Part model, mm, in its own coordinate system. A direction names the side the tool comes from. Round coordinates to 2 decimals unless told otherwise and drop trailing zeros. Write each loop counter-clockwise with the first axis right and the second up, starting at its lowest first coordinate (ties: lowest second). Pieces come first, ordered by that corner, then holes. Notation, with made-up numbers: M 64.25,-20.5 L 106.25,-20.5 A32 ccw 106.25,10.5 Z; hole C 15,-36 d10. An arc over 180 degrees is marked long. Use a Markdown table: item, result. Add a question column.
1) Two-plate mould, pull along Z, no slides. Class faces 1 (the face through (100.487, 3.479, -4.305)), 2 (the face through (113, 2, -64)), 3 (the face through (-14.5, 35, -21)): released by +Z, released by -Z, zero draft, split by the parting line, or undercut.
2) Which spindle directions (+Z, -Z, +X, -X, +Y, -Y) get a long thin tool onto all of the face, cutting with end or side? Do faces 4 (the face through (113, 2, 18)), 5 (the face through (-1.2, 52.5, -25.5)), 6 (the face through (41.974, 0.986, -4.109)), 7 (the face through (113, 2, 29)). Say none if no direction does.
3) Slice it at B-B on z = -26.7. Write the cut outline in (x, y), plus the area to 3 significant figures.
4) Drop flat-ended pins along their axis: P1, Ø1.8, axis at x = 98.5, z = -68.5, coming from the -Y side; P2, Ø4, axis at x = 20, y = 47, coming from the +Z side; P3, Ø5.5, axis at y = 2, z = 22.5, coming from the -X side; P4, Ø1, axis at y = 20.5, z = -43.5, coming from the -X side. Give the stop position or say it passes through.
5) Wall check: probe 1 along X at (y, z) = (51, -3); probe 2 along Z at (x, y) = (99, 4.25); probe 3 along X at (y, z) = (0.55, -67.5). Give the ranges that are in metal, low to high.
6) Slice it at D-D on y = 23. Write the cut outline in (x, z).
7) Slice it at A-A on x = 10. Write the cut outline in (y, z), plus the area to 3 significant figures.
8) Slice it at C-C on x = 25. Write the cut outline in (y, z).
```python
from build123d import *

# Parameters (mm, degrees)
SKETCH_1_W               = 4
SKETCH_1_H               = 42
SKETCH_1_W_2             = 29
SKETCH_1_W_3             = 16
EXTRUDE_2_DEPTH          = 90
CUT_EXTRUDE_3_DEPTH      = 30
CUT_EXTRUDE_3_DEPTH_BACK = 1
SKETCH_1_6_W             = 29
SKETCH_1_6_H             = 42
SKETCH_7_W               = 77
SKETCH_7_H               = 115
CUT_EXTRUDE_5_DEPTH      = 85
SKETCH_8_W               = 49
SKETCH_8_H               = 42
CUT_EXTRUDE_6_DEPTH      = 55
SKETCH_11_R              = 1.5
CUT_EXTRUDE_9_DEPTH      = 6
SKETCH_14_R              = 3
CUT_EXTRUDE_11_DEPTH     = 2
SKETCH_18_W              = 49
SKETCH_18_H              = 42
EXTRUDE_3_DEPTH          = 20
SKETCH_19_W              = 29
SKETCH_19_H              = 42
CUT_EXTRUDE_14_DEPTH     = 20
SKETCH_20_R              = 1.5
CUT_EXTRUDE_15_DEPTH     = 141.289878466
SKETCH_21_R              = 2.75
CUT_EXTRUDE_16_DEPTH     = 2.5
SKETCH_25_W              = 4
SKETCH_25_H              = 42
CUT_EXTRUDE_18_DEPTH     = 20
SKETCH_26_W              = 11
SKETCH_26_H              = 11
EXTRUDE_4_DEPTH          = 5
SKETCH_28_R              = 3
CUT_EXTRUDE_19_DEPTH     = 151.639470259


with BuildPart() as part:
    # 草图1 → 凸台-拉伸2 (new body)
    with BuildSketch(Plane(origin=(0, 0, 0), x_dir=(1, 0, 0), z_dir=(0, 1, 0))):
        with Locations((-16.5, 21)):
            Rectangle(SKETCH_1_W, SKETCH_1_H)
        with Locations((0, 21)):
            Rectangle(SKETCH_1_W_2, SKETCH_1_H)
        with Locations((22.5, 21)):
            Rectangle(SKETCH_1_W_3, SKETCH_1_H)
        with Locations((32.5, 21)):
            Rectangle(SKETCH_1_W, SKETCH_1_H)
        Polygon((30.5, 75), (30.5, 42), (34.5, 42), (34.5, 0), (30.5, 0), (30.5, -40), (107.5, -40), (107.5, 75), align=None)
    extrude(amount=EXTRUDE_2_DEPTH)

    # 草图1<6> → 切除-拉伸3 (cut, two sides: drawn at the far end of the back side and taken through both)
    with BuildSketch(Plane(origin=(0, 0, 0), x_dir=(1, 0, 0), z_dir=(0, 1, 0)).offset(-CUT_EXTRUDE_3_DEPTH_BACK)):
        with Locations((0, 21)):
            Rectangle(SKETCH_1_6_W, SKETCH_1_6_H)
    extrude(amount=CUT_EXTRUDE_3_DEPTH + CUT_EXTRUDE_3_DEPTH_BACK, mode=Mode.SUBTRACT)

    # 草图7 → 切除-拉伸5 (cut)
    with BuildSketch(Plane(origin=(0, 90, 0), x_dir=(1, 0, 0), z_dir=(0, 1, 0))):
        with Locations((69, 17.5)):
            Rectangle(SKETCH_7_W, SKETCH_7_H)
    extrude(amount=-CUT_EXTRUDE_5_DEPTH, mode=Mode.SUBTRACT)

    # 草图8 → 切除-拉伸6 (cut)
    with BuildSketch(Plane(origin=(0, 90, 0), x_dir=(1, 0, 0), z_dir=(0, 1, 0))):
        with Locations((6, 21)):
            Rectangle(SKETCH_8_W, SKETCH_8_H)
    extrude(amount=-CUT_EXTRUDE_6_DEPTH, mode=Mode.SUBTRACT)

    # 草图11 → 切除-拉伸9 (cut)
    with BuildSketch(Plane.XZ):
        with Locations(Location((39, 33, 0), (0, 0, 270))):
            Circle(SKETCH_11_R)
        with Locations(Location((99, 33, 0), (0, 0, 270))):
            Circle(SKETCH_11_R)
        with Locations(Location((39, -4.5, 0), (0, 0, 270))):
            Circle(SKETCH_11_R)
        with Locations(Location((99, -4.5, 0), (0, 0, 270))):
            Circle(SKETCH_11_R)
        with Locations(Location((99, -67.5, 0), (0, 0, 270))):
            Circle(SKETCH_11_R)
        with Locations(Location((39, -67.5, 0), (0, 0, 270))):
            Circle(SKETCH_11_R)
    extrude(amount=-CUT_EXTRUDE_9_DEPTH, mode=Mode.SUBTRACT)

    # 草图14 → 切除-拉伸11 (cut)
    with BuildSketch(Plane.XZ):
        with Locations(Location((39, 33, 0), (0, 0, 270))):
            Circle(SKETCH_14_R)
        with Locations(Location((99, 33, 0), (0, 0, 270))):
            Circle(SKETCH_14_R)
        with Locations(Location((39, -4.5, 0), (0, 0, 270))):
            Circle(SKETCH_14_R)
        with Locations(Location((99, -4.5, 0), (0, 0, 270))):
            Circle(SKETCH_14_R)
        with Locations(Location((39, -67.5, 0), (0, 0, 270))):
            Circle(SKETCH_14_R)
        with Locations(Location((99, -67.5, 0), (0, 0, 270))):
            Circle(SKETCH_14_R)
    extrude(amount=-CUT_EXTRUDE_11_DEPTH, mode=Mode.SUBTRACT)

    # 草图18 → 凸台-拉伸3 (add)
    with BuildSketch(Plane(origin=(0, 35, 0), x_dir=(1, 0, 0), z_dir=(0, 1, 0))):
        with Locations((6, 21)):
            Rectangle(SKETCH_18_W, SKETCH_18_H)
    extrude(amount=EXTRUDE_3_DEPTH)

    # 草图19 → 切除-拉伸14 (cut)
    with BuildSketch(Plane.XZ.offset(-30)):
        with Locations((0, -21)):
            Rectangle(SKETCH_19_W, SKETCH_19_H)
    extrude(amount=-CUT_EXTRUDE_14_DEPTH, mode=Mode.SUBTRACT)

    # 草图20 → 切除-拉伸15 (cut, through all)
    with BuildSketch(Plane.XZ.offset(-50)):
        with Locations(Location((-10, -3, 0), (0, 0, 270))):
            Circle(SKETCH_20_R)
        with Locations(Location((10, -3, 0), (0, 0, 270))):
            Circle(SKETCH_20_R)
        with Locations(Location((0, -26.7, 0), (0, 0, 270))):
            Circle(SKETCH_20_R)
    extrude(amount=-CUT_EXTRUDE_15_DEPTH, mode=Mode.SUBTRACT)

    # 草图21 → 切除-拉伸16 (cut)
    with BuildSketch(Plane(origin=(0, 55, 0), x_dir=(1, 0, 0), z_dir=(0, 1, 0))):
        with Locations(Location((0, 26.7, 0), (0, 0, 270))):
            Circle(SKETCH_21_R)
        with Locations(Location((-10, 3, 0), (0, 0, 270))):
            Circle(SKETCH_21_R)
        with Locations(Location((10, 3, 0), (0, 0, 270))):
            Circle(SKETCH_21_R)
    extrude(amount=-CUT_EXTRUDE_16_DEPTH, mode=Mode.SUBTRACT)

    # 草图25 → 切除-拉伸18 (cut)
    with BuildSketch(Plane.XZ):
        with Locations((-16.5, -21)):
            Rectangle(SKETCH_25_W, SKETCH_25_H)
    extrude(amount=-CUT_EXTRUDE_18_DEPTH, mode=Mode.SUBTRACT)

    # 草图26 → 凸台-拉伸4 (add)
    with BuildSketch(Plane.XZ):
        with Locations((25, 23.5)):
            Rectangle(SKETCH_26_W, SKETCH_26_H)
        with Locations((113, 23.5)):
            Rectangle(SKETCH_26_W, SKETCH_26_H)
        with Locations((25, -58.5)):
            Rectangle(SKETCH_26_W, SKETCH_26_H)
        with Locations((113, -58.5)):
            Rectangle(SKETCH_26_W, SKETCH_26_H)
    extrude(amount=-EXTRUDE_4_DEPTH)

    # 草图28 → 切除-拉伸19 (cut, through all)
    with BuildSketch(Plane.XZ):
        with Locations(Location((25, 23.5, 0), (0, 0, 270))):
            Circle(SKETCH_28_R)
        with Locations(Location((113, 23.5, 0), (0, 0, 270))):
            Circle(SKETCH_28_R)
        with Locations(Location((25, -58.5, 0), (0, 0, 270))):
            Circle(SKETCH_28_R)
        with Locations(Location((113, -58.5, 0), (0, 0, 270))):
            Circle(SKETCH_28_R)
    extrude(amount=-CUT_EXTRUDE_19_DEPTH, mode=Mode.SUBTRACT)


solid = part.part
```
Entries:
| question | item | result |
|---|---|---|
| 1 | face 1 | undercut |
| 1 | face 2 | released by -Z |
| 1 | face 3 | zero draft |
| 2 | face 4 | +X, +Y, -Y |
| 2 | face 5 | +Y |
| 2 | face 6 | -Y |
| 2 | face 7 | +Z, +X, +Y, -Y |
| 3 | outline | M -18.5,20 L -14.5,20 L -14.5,50 L -1.5,50 L -1.5,52.5 L -2.75,52.5 L -2.75,55 L -18.5,55 Z; M 1.5,50 L 14.5,50 L 14.5,0 L 107.5,0 L 107.5,5 L 30.5,5 L 30.5,55 L 2.75,55 L 2.75,52.5 L 1.5,52.5 Z |
| 3 | area | 1,530 mm^2 |
| 4 | P1 | stops at y = 2 |
| 4 | P2 | stops at z = 0 |
| 4 | P3 | stops at x = 19.5 |
| 4 | P4 | passes through |
| 5 | probe 1 | x = -18.5 to -11.5, -8.5 to 8.5, 11.5 to 30.5 |
| 5 | probe 2 | z = -75 to -69, -66 to -6, -3 to 31.5, 34.5 to 40 |
| 5 | probe 3 | x = 30.5 to 36, 42 to 96, 102 to 107.5 |
| 6 | outline | M -18.5,-42 L -14.5,-42 L -14.5,0 L -18.5,0 Z; M 14.5,-42 L 30.5,-42 L 30.5,0 L 14.5,0 Z |
| 7 | outline | M 50,-42 L 55,-42 L 55,-5.75 L 52.5,-5.75 L 52.5,-4.5 L 50,-4.5 Z; M 50,-1.5 L 52.5,-1.5 L 52.5,-0.25 L 55,-0.25 L 55,0 L 50,0 Z |
| 7 | area | 189 mm^2 |
| 8 | outline | M 0,-64 L 5,-64 L 5,-61.5 L 0,-61.5 Z; M 0,-55.5 L 5,-55.5 L 5,-53 L 0,-53 Z; M 0,-42 L 55,-42 L 55,0 L 0,0 Z; M 0,18 L 5,18 L 5,20.5 L 0,20.5 Z; M 0,26.5 L 5,26.5 L 5,29 L 0,29 Z |
